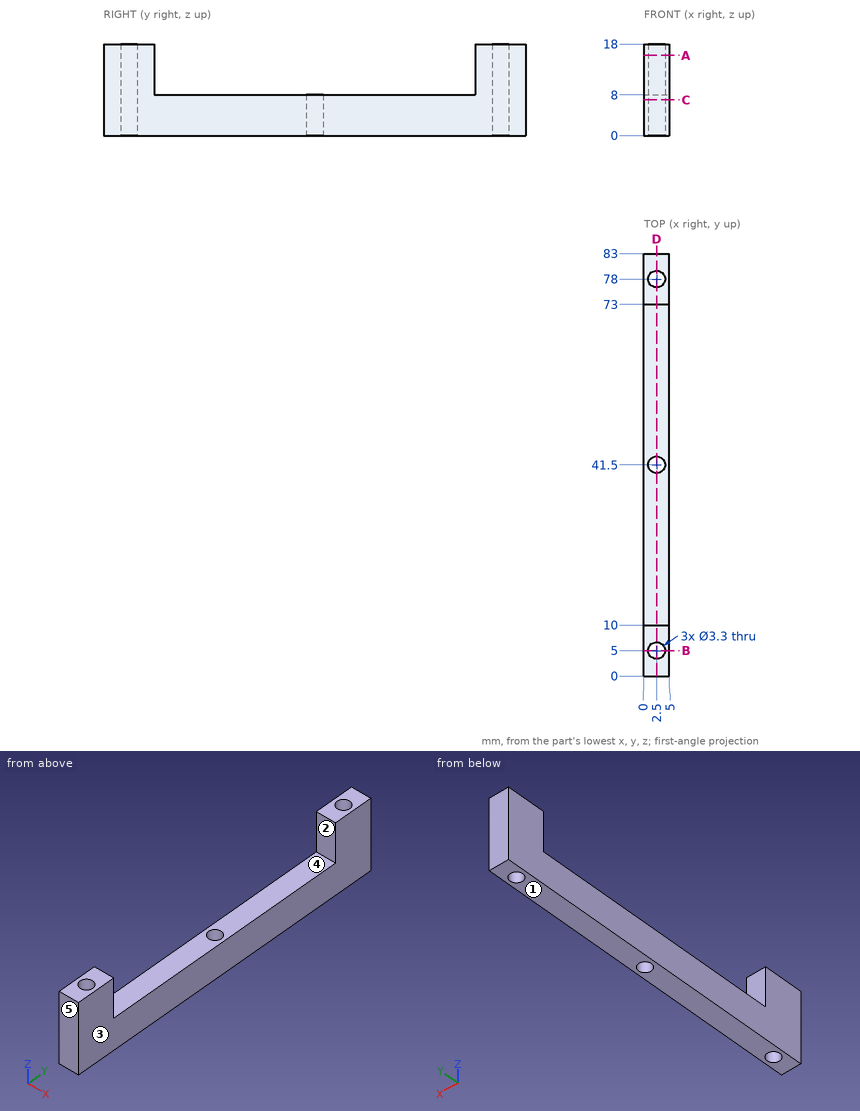
Drawing for the job (mm, zero at the part's lowest x, y, z). A direction names the side the tool comes from. Coordinates: 2 decimals unless noted, no trailing zeros. Order: outer loops, then holes, each group sorted by start corner. A loop starts at its lowest first (then second) coordinate and runs counter-clockwise, first axis right, second up.
Item 1: Band-saw the part on D-D on x = 2.5. List the corners of the cut face in (y, z), plus the area to 3 significant figures.
Check sheet entries:
outline: (0, 0) - (3.35, 0) - (3.35, 18) - (0, 18) - close; (6.65, 0) - (39.85, 0) - (39.85, 8) - (10, 8) - (10, 18) - (6.65, 18) - close; (43.15, 0) - (76.35, 0) - (76.35, 18) - (73, 18) - (73, 8) - (43.15, 8) - close; (79.65, 0) - (83, 0) - (83, 18) - (79.65, 18) - close
area: 719 mm2
Item 2: Pin check, flat tip, straight feed: pin 1 Ø1.5 at (x, y) = (2, 27.5) entering from +Z. Stop position of the tip, or through.
Check sheet entries:
pin 1: stops at z = 8
Item 3: Band-saw the part on B-B on y = 5. List the corners of the cut face in (x, z).
Check sheet entries:
outline: (0, 0) - (0.85, 0) - (0.85, 18) - (0, 18) - close; (4.15, 0) - (5, 0) - (5, 18) - (4.15, 18) - close
Item 4: 3-axis set-ups, long thin cutter, end or side, ignore diameter. For the marked faces 1 and 2: which of +Z, -Z, +X, -X, +Y, -Y reach the whole face in a straight line?
Check sheet entries:
face 1: -Z, +X, -X, +Y, -Y
face 2: +Z, +X, -X
Item 5: Band-saw the part on C-C on z = 7. List the corners of the cut face in (x, y).
Check sheet entries:
outline: (0, 0) - (5, 0) - (5, 83) - (0, 83) - close; hole circle Ø3.3 at (2.5, 5); hole circle Ø3.3 at (2.5, 41.5); hole circle Ø3.3 at (2.5, 78)
Item 6: Two-plate mould, pull along Y, no slides. Class the marked faces 3, 4 and 5: +Y half, -Y half, draft (parallel to the pull), parting line (faces both ways), or undercut.
Check sheet entries:
face 3: draft
face 4: undercut
face 5: -Y half
Item 7: Drill centre lines: L1, parallel to Y at x = 2.5, z = 12; L2, parallel to Y at x = 2.5, z = 4.5; L3, parallel to X at y = 78, z = 13. Where is each one in solid material? Low to high.
Check sheet entries:
L1: y = 0 to 3.35, 6.65 to 10, 73 to 76.35, 79.65 to 83
L2: y = 0 to 3.35, 6.65 to 39.85, 43.15 to 76.35, 79.65 to 83
L3: x = 0 to 0.85, 4.15 to 5
Item 8: Band-saw the part on A-A on z = 15.75. List the corners of the cut face in (x, y).
Check sheet entries:
outline: (0, 0) - (5, 0) - (5, 10) - (0, 10) - close; (0, 73) - (5, 73) - (5, 83) - (0, 83) - close; hole circle Ø3.3 at (2.5, 5); hole circle Ø3.3 at (2.5, 78)
